Part model, mm, in its own coordinate system. A direction names the side the tool comes from. Round coordinates to 2 decimals unless told otherwise and drop trailing zeros. Loops run counter-clockwise (first coordinate to the right, second up) from the corner with the lowest first, then second, coordinate; pieces in that order, holes last. Notation, with made-up numbers: M 7.25,-37.5 L 52.25,-37.5 A8 ccw 52.25,-31.5 Z; hole C 17.5,82 d1. An arc over 180 degrees is marked long. Write each question's results on one line, items separated by ' | '.
from build123d import *

# Parameters (mm, degrees)
SKETCH1_R           = 19.61817075
BOSS_EXTRUDE1_DEPTH = 3.175
FILLET1_R           = 25.4
SKETCH2_R           = 15.875
BOSS_EXTRUDE2_DEPTH = 12.7
CUT_EXTRUDE3_START  = -6.35
SKETCH5_R           = 15.875
CUT_EXTRUDE3_DEPTH  = 6.35
SKETCH3_R           = 3.175
CUT_EXTRUDE1_DEPTH  = 12.7
SKETCH4_R           = 3.175
CUT_EXTRUDE2_DEPTH  = 12.7
CUT_EXTRUDE4_START  = -23.876
SKETCH7_R           = 22.225
SKETCH7_R_2         = 15.875
CUT_EXTRUDE4_DEPTH  = 23.876


with BuildPart() as part:
    # Sketch1 → Boss-Extrude1 (new body)
    with BuildSketch(Plane.XY):
        with BuildLine():
            ThreePointArc((44.489667751, 31.288325121), (28.726604254, 41.946482698), (22.64318373, 59.97597211))
            ThreePointArc((22.64318373, 59.97597211), (16.800558188, 80.054274158), (1.097123352, 93.862844712))
            Line((1.097123352, 93.862844712), (1.097123352, 122.797032487))
            Line((1.097123352, 122.797032487), (-30.652876648, 122.797032487))
            Line((-30.652876648, 122.797032487), (-30.652876648, 93.862844712))
            ThreePointArc((-30.652876648, 93.862844712), (-46.356311483, 80.054274158), (-52.198937025, 59.97597211))
            ThreePointArc((-52.198937025, 59.97597211), (-58.282357549, 41.946482698), (-74.045421046, 31.288325121))
            ThreePointArc((-74.045421046, 31.288325121), (-89.694055432, 20.335242519), (-97.327876648, 2.82597211))
            Line((-97.327876648, 2.82597211), (-97.327876648, -35.27402789))
            Line((-97.327876648, -35.27402789), (-34.257381722, -35.27402789))
            Line((-34.257381722, -35.27402789), (-34.257381722, -22.57402789))
            add(Edge.make_bspline(
                [(4.701628427, -22.57402789), (4.701628427, 9.595471172), (-14.777876648, 9.595471172), (-34.257381722, 9.595471172), (-34.257381722, -22.57402789)],
                knots=[1.570796327, 1.570796327, 1.570796327, 3.141592654, 3.141592654, 4.71238898, 4.71238898, 4.71238898], degree=2, weights=[1, 0.707106781, 1, 0.707106781, 1]))
            Line((4.701628427, -22.57402789), (4.701628427, -35.27402789))
            Line((4.701628427, -35.27402789), (67.772123352, -35.27402789))
            Line((67.772123352, -35.27402789), (67.772123352, 2.82597211))
            ThreePointArc((67.772123352, 2.82597211), (60.138302137, 20.335242519), (44.489667751, 31.288325121))
        make_face()
        with Locations((-14.777876648, 59.97597211)):
            Circle(SKETCH1_R, mode=Mode.SUBTRACT)
    extrude(amount=BOSS_EXTRUDE1_DEPTH)

    # Fillet1
    fillet1_edges = [part.edges().sort_by_distance(p)[0] for p in [
        (-30.652876648, 93.862844712, 1.5875),
        (1.097123352, 93.862844712, 1.5875),
    ]]
    fillet(fillet1_edges, radius=FILLET1_R)

    # Sketch2 → Boss-Extrude2 (add)
    with BuildSketch(Plane.XY.offset(3.175)):
        with BuildLine():
            Line((1.097123352, 107.334815022), (1.097123352, 122.797032487))
            Line((1.097123352, 122.797032487), (-30.652876648, 122.797032487))
            Line((-30.652876648, 122.797032487), (-30.652876648, 107.334815022))
            ThreePointArc((-30.652876648, 107.334815022), (-32.933121295, 96.816406756), (-39.364444557, 88.186545274))
            ThreePointArc((-39.364444557, 88.186545274), (-48.83952078, 75.47242844), (-52.198937025, 59.97597211))
            ThreePointArc((-52.198937025, 59.97597211), (-58.282357549, 41.946482698), (-74.045421046, 31.288325121))
            ThreePointArc((-74.045421046, 31.288325121), (-89.694055432, 20.335242519), (-97.327876648, 2.82597211))
            Line((-97.327876648, 2.82597211), (-97.327876648, -35.27402789))
            Line((-97.327876648, -35.27402789), (-34.257381722, -35.27402789))
            Line((-34.257381722, -35.27402789), (-34.257381722, -22.57402789))
            add(Edge.make_bspline(
                [(4.701628427, -22.57402789), (4.701628427, 9.595471172), (-14.777876648, 9.595471172), (-34.257381722, 9.595471172), (-34.257381722, -22.57402789)],
                knots=[1.570796327, 1.570796327, 1.570796327, 3.141592654, 3.141592654, 4.71238898, 4.71238898, 4.71238898], degree=2, weights=[1, 0.707106781, 1, 0.707106781, 1]))
            Line((4.701628427, -22.57402789), (4.701628427, -35.27402789))
            Line((4.701628427, -35.27402789), (67.772123352, -35.27402789))
            Line((67.772123352, -35.27402789), (67.772123352, 2.82597211))
            ThreePointArc((67.772123352, 2.82597211), (60.138302137, 20.335242519), (44.489667751, 31.288325121))
            ThreePointArc((44.489667751, 31.288325121), (28.726604254, 41.946482698), (22.64318373, 59.97597211))
            ThreePointArc((22.64318373, 59.97597211), (19.283767485, 75.47242844), (9.808691261, 88.186545274))
            ThreePointArc((9.808691261, 88.186545274), (3.377368, 96.816406756), (1.097123352, 107.334815022))
        make_face()
        with Locations((-14.777876648, 59.97597211)):
            Circle(SKETCH2_R, mode=Mode.SUBTRACT)
    extrude(amount=BOSS_EXTRUDE2_DEPTH)

    # Sketch5 → Cut-Extrude3 (cut)
    with BuildSketch(Plane.XY.offset(15.875).offset(CUT_EXTRUDE3_START)):
        with BuildLine():
            Line((1.097123352, 107.334815022), (1.097123352, 122.797032487))
            Line((1.097123352, 122.797032487), (-30.652876648, 122.797032487))
            Line((-30.652876648, 122.797032487), (-30.652876648, 107.334815022))
            ThreePointArc((-30.652876648, 107.334815022), (-32.933121295, 96.816406756), (-39.364444557, 88.186545274))
            ThreePointArc((-39.364444557, 88.186545274), (-48.83952078, 75.47242844), (-52.198937025, 59.97597211))
            ThreePointArc((-52.198937025, 59.97597211), (-58.282357549, 41.946482698), (-74.045421046, 31.288325121))
            ThreePointArc((-74.045421046, 31.288325121), (-89.694055432, 20.335242519), (-97.327876648, 2.82597211))
            Line((-97.327876648, 2.82597211), (-97.327876648, -35.27402789))
            Line((-97.327876648, -35.27402789), (-34.257381722, -35.27402789))
            Line((-34.257381722, -35.27402789), (-34.257381722, -22.57402789))
            add(Edge.make_bspline(
                [(4.701628427, -22.57402789), (4.701628427, 9.595471172), (-14.777876648, 9.595471172), (-34.257381722, 9.595471172), (-34.257381722, -22.57402789)],
                knots=[1.570796327, 1.570796327, 1.570796327, 3.141592654, 3.141592654, 4.71238898, 4.71238898, 4.71238898], degree=2, weights=[1, 0.707106781, 1, 0.707106781, 1]))
            Line((4.701628427, -22.57402789), (4.701628427, -35.27402789))
            Line((4.701628427, -35.27402789), (67.772123352, -35.27402789))
            Line((67.772123352, -35.27402789), (67.772123352, 2.82597211))
            ThreePointArc((67.772123352, 2.82597211), (60.138302137, 20.335242519), (44.489667751, 31.288325121))
            ThreePointArc((44.489667751, 31.288325121), (28.726604254, 41.946482698), (22.64318373, 59.97597211))
            ThreePointArc((22.64318373, 59.97597211), (19.283767485, 75.47242844), (9.808691261, 88.186545274))
            ThreePointArc((9.808691261, 88.186545274), (3.377368, 96.816406756), (1.097123352, 107.334815022))
        make_face()
        with Locations((-14.777876648, 59.97597211)):
            Circle(SKETCH5_R, mode=Mode.SUBTRACT)
    extrude(amount=CUT_EXTRUDE3_DEPTH, mode=Mode.SUBTRACT)

    # Sketch3 → Cut-Extrude1 (cut)
    with BuildSketch(Plane.XZ.offset(35.27402789)):
        with Locations((-50.025005454, 4.7625)):
            Circle(SKETCH3_R)
        with Locations((-81.560252916, 4.7625)):
            Circle(SKETCH3_R)
        with Locations(Location((20.469252158, 4.7625, 0), (0, 0, 180))):
            Circle(SKETCH3_R)
        with Locations(Location((52.004499621, 4.7625, 0), (0, 0, 180))):
            Circle(SKETCH3_R)
    extrude(amount=-CUT_EXTRUDE1_DEPTH, mode=Mode.SUBTRACT)

    # Sketch4 → Cut-Extrude2 (cut)
    with BuildSketch(Plane(origin=(0, 122.797032487, 0), x_dir=(1, 0, 0), z_dir=(0, 1, 0))):
        with Locations(Location((-22.715376648, -4.7625, 0), (0, 0, 270))):
            Circle(SKETCH4_R)
        with Locations(Location((-6.840376648, -4.7625, 0), (0, 0, 270))):
            Circle(SKETCH4_R)
    extrude(amount=-CUT_EXTRUDE2_DEPTH, mode=Mode.SUBTRACT)

    # Sketch7 → Cut-Extrude4 (cut)
    with BuildSketch(Plane.XY.offset(9.525).offset(CUT_EXTRUDE4_START)):
        with Locations((-14.777876648, 59.97597211)):
            Circle(SKETCH7_R)
        with Locations((-14.777876648, 59.97597211)):
            Circle(SKETCH7_R_2, mode=Mode.SUBTRACT)
    extrude(amount=CUT_EXTRUDE4_DEPTH, mode=Mode.SUBTRACT)


solid = part.part
Item 1: Band-saw the part on B-B on x = 34. Give the cut face in (y, z) (3 decimals), and give its area (3 significant figures).
Filled sheet:
outline: M -35.274,0 L 36.589,0 L 36.589,9.525 L -35.274,9.525 Z | area: 684 mm^2
Item 2: Wall check: L1, parallel to X at y = 110.5, z = 5; L2, parallel to Y at x = -17, z = 5; L3, parallel to X at y = 75, z = 3.5. Give the ranges that are in metal, low to high.
Filled sheet:
L1: -30.65 to -25.88, -19.55 to -10.01, -3.67 to 1.1 | L2: 9.39 to 37.86, 82.09 to 122.8 | L3: -49.05 to -31.16, 1.6 to 19.49
Item 3: Band-saw the part on D-D on x = -44.5. Give the cut face in (y, z) (3 decimals), and give its area (3 significant figures).
Filled sheet:
outline: M -35.274,0 L 82.712,0 L 82.712,9.525 L -35.274,9.525 Z | area: 1,120 mm^2
Item 4: Band-saw the part on C-C on y = 23. Give the cut face in (x, z) (3 decimals).
Filled sheet:
outline: M -87.277,0 L 57.721,0 L 57.721,9.525 L -87.277,9.525 Z
Item 5: Drop flat-ended pins along their axis: P1, Ø3, axis at x = -49, z = 4.5, coming from the -Y side; P2, Ø3, axis at x = -7.5, z = 3, coming from the +Y side; P3, Ø5, axis at x = -22.72, z = 4.76, coming from the +Y side; P4, Ø1, axis at y = 50, z = 8.5, coming from the +X side. Give the stop position or say it passes through.
Filled sheet:
P1: y = -22.57 | P2: y = 122.8 | P3: y = 110.1 | P4: x = 24.55
Item 6: Two-plate mould, pull along X, no slides. Class faces 1 (the flat face through (-16, 27, 9.525)), 2 (the flat face through (4.702, -29, 5)), 3 (the cylindrical face through (-58.12, 42.16, 4.7)): +X half, -X half, draft (parallel to the pull), parting line (faces both ways), or undercut.
Filled sheet:
face 1: draft | face 2: undercut | face 3: -X half
Item 7: Which spindle directions (+Z, -Z, +X, -X, +Y, -Y) get a long thin tool onto all of the face, cutting with end or side? Do faces 4 (the flat face through (-23, 110.097, 5)), 5 (the flat face through (21, -22.574, 5)), 6 (the flat face through (-30.653, 115, 5)), 7 (the flat face through (1.097, 115, 5)). Say none if no direction does.
Filled sheet:
face 4: +Y | face 5: -Y | face 6: +Z, -Z, -X, +Y | face 7: +Z, -Z, +X, +Y
Item 8: Band-saw the part on A-A on y = 46.5. Give the cut face in (x, z) (3 decimals).
Filled sheet:
outline: M -55.425,0 L -32.451,0 L -32.451,9.525 L -55.425,9.525 Z; M 2.896,0 L 25.869,0 L 25.869,9.525 L 2.896,9.525 Z
